from build123d import *

# Parameters (mm, degrees)
F0_R     = 9.4
F1_DEPTH = 3


with BuildPart() as f1:
    # F0 (on Front) → F1 (new body)
    with BuildSketch(Plane.XZ):
        with BuildLine():
            ThreePointArc((-5.1, -8.833459), (-3.333588, -10.15167), (-1.922689, -11.844968))
            ThreePointArc((-1.922689, -11.844968), (-0.788709, -14.298908), (-0.4, -16.974098))
            ThreePointArc((-0.4, -16.974098), (0.966541, -22.074098), (4.7, -25.807557))
            ThreePointArc((4.7, -25.807557), (8.140639, -29.248196), (9.4, -33.948196))
            ThreePointArc((9.4, -33.948196), (10.766541, -39.048196), (14.5, -42.781655))
            ThreePointArc((14.5, -42.781655), (17.940639, -46.222294), (19.2, -50.922294))
            ThreePointArc((19.2, -50.922294), (20.566541, -56.022294), (24.3, -59.755753))
            ThreePointArc((24.3, -59.755753), (27.740639, -63.196392), (29, -67.896392))
            ThreePointArc((29, -67.896392), (30.366541, -72.996392), (34.1, -76.729851))
            ThreePointArc((34.1, -76.729851), (37.540639, -80.17049), (38.8, -84.87049))
            ThreePointArc((38.8, -84.87049), (40.166541, -89.97049), (43.9, -93.703949))
            ThreePointArc((43.9, -93.703949), (47.340639, -97.144587), (48.6, -101.844587))
            ThreePointArc((48.6, -101.844587), (48.341601, -104.033451), (47.580612, -106.101974))
            ThreePointArc((47.580612, -106.101974), (51.984159, -111.72104), (58.8, -113.844587))
            Line((58.8, -113.844587), (98, -113.844587))
            ThreePointArc((98, -113.844587), (104.815841, -111.72104), (109.219388, -106.101974))
            ThreePointArc((109.219388, -106.101974), (108.458399, -104.033451), (108.2, -101.844587))
            ThreePointArc((108.2, -101.844587), (106.833459, -96.744587), (103.1, -93.011128))
            ThreePointArc((103.1, -93.011128), (99.659361, -89.57049), (98.4, -84.87049))
            ThreePointArc((98.4, -84.87049), (97.033459, -79.77049), (93.3, -76.03703))
            ThreePointArc((93.3, -76.03703), (89.859361, -72.596392), (88.6, -67.896392))
            ThreePointArc((88.6, -67.896392), (87.233459, -62.796392), (83.5, -59.062933))
            ThreePointArc((83.5, -59.062933), (80.059361, -55.622294), (78.8, -50.922294))
            ThreePointArc((78.8, -50.922294), (77.433459, -45.822294), (73.7, -42.088835))
            ThreePointArc((73.7, -42.088835), (70.259361, -38.648196), (69, -33.948196))
            ThreePointArc((69, -33.948196), (67.633459, -28.848196), (63.9, -25.114737))
            ThreePointArc((63.9, -25.114737), (60.459361, -21.674098), (59.2, -16.974098))
            ThreePointArc((59.2, -16.974098), (57.833459, -11.874098), (54.1, -8.140639))
            ThreePointArc((54.1, -8.140639), (50.659361, -4.7), (49.4, 0))
            ThreePointArc((49.4, 0), (49.658399, 2.188863), (50.419388, 4.257386))
            ThreePointArc((50.419388, 4.257386), (46.015841, 9.876453), (39.2, 12))
            Line((39.2, 12), (0, 12))
            ThreePointArc((0, 12), (-6.815841, 9.876453), (-11.219388, 4.257386))
            ThreePointArc((-11.219388, 4.257386), (-10.2, 0), (-11.219388, -4.257386))
            ThreePointArc((-11.219388, -4.257386), (-10.392305, -6), (-9.296699, -7.587582))
            ThreePointArc((-9.296699, -7.587582), (-7.12481, -7.962807), (-5.1, -8.833459))
        make_face()
        with BuildLine():
            ThreePointArc((56.877311, -89.99962), (39.988709, -82.1953), (58.4, -84.87049))
            ThreePointArc((58.4, -84.87049), (58.011291, -87.545679), (56.877311, -89.99962))
        make_face(mode=Mode.SUBTRACT)
        with Locations((39.2, -67.896392)):
            Circle(F0_R, mode=Mode.SUBTRACT)
        with Locations((58.8, -101.844587)):
            Circle(F0_R, mode=Mode.SUBTRACT)
        with Locations((78.4, -101.844587)):
            Circle(F0_R, mode=Mode.SUBTRACT)
        with BuildLine():
            ThreePointArc((78, -84.87049), (71.27519, -93.88178), (60.722689, -89.99962))
            ThreePointArc((60.722689, -89.99962), (65.92481, -75.859199), (78, -84.87049))
        make_face(mode=Mode.SUBTRACT)
        with Locations((98, -101.844587)):
            Circle(F0_R, mode=Mode.SUBTRACT)
        with Locations((88.2, -84.87049)):
            Circle(F0_R, mode=Mode.SUBTRACT)
        with Locations((58.8, -67.896392)):
            Circle(F0_R, mode=Mode.SUBTRACT)
        with Locations((78.4, -67.896392)):
            Circle(F0_R, mode=Mode.SUBTRACT)
        with Locations((29.4, -50.922294)):
            Circle(F0_R, mode=Mode.SUBTRACT)
        with Locations((49, -50.922294)):
            Circle(F0_R, mode=Mode.SUBTRACT)
        with Locations((19.6, -33.948196)):
            Circle(F0_R, mode=Mode.SUBTRACT)
        with Locations((39.2, -33.948196)):
            Circle(F0_R, mode=Mode.SUBTRACT)
        with BuildLine():
            ThreePointArc((1.922689, -11.844968), (12.47519, -7.962807), (19.2, -16.974098))
            ThreePointArc((19.2, -16.974098), (7.12481, -25.985389), (1.922689, -11.844968))
        make_face(mode=Mode.SUBTRACT)
        Circle(F0_R, mode=Mode.SUBTRACT)
        with Locations((29.4, -16.974098)):
            Circle(F0_R, mode=Mode.SUBTRACT)
        with BuildLine():
            ThreePointArc((53.7, -25.114737), (40.859361, -21.674098), (44.3, -8.833459))
            ThreePointArc((44.3, -8.833459), (57.140639, -12.274098), (53.7, -25.114737))
        make_face(mode=Mode.SUBTRACT)
        with Locations((19.6, 0)):
            Circle(F0_R, mode=Mode.SUBTRACT)
        with Locations((39.2, 0)):
            Circle(F0_R, mode=Mode.SUBTRACT)
        with Locations((68.6, -50.922294)):
            Circle(F0_R, mode=Mode.SUBTRACT)
        with Locations((58.8, -33.948196)):
            Circle(F0_R, mode=Mode.SUBTRACT)
    extrude(amount=F1_DEPTH)


solid = f1.part
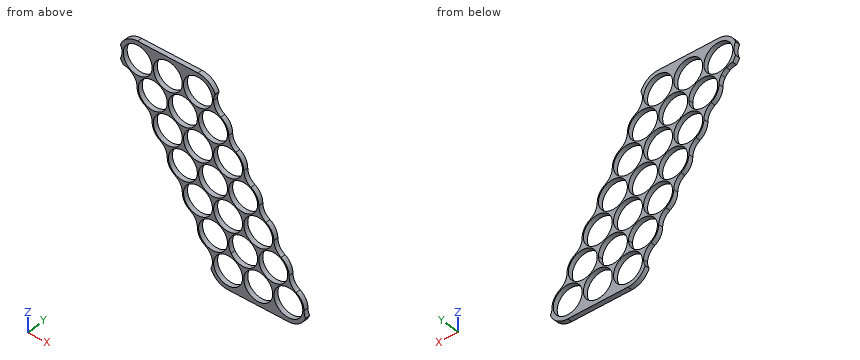
Design review of the part built by this model. Coordinates are the model's own, in mm. Coordinates: 2 decimals unless noted, no trailing zeros. Use one line per item in the form item = value.
(1) For line 1 along X through (y, z) = (-1.85, -34); line 2 along X through (y, z) = (-2.4, -12); line 3 along Z through (x, y) = (90.5, -2.2), list the stretches that pass through material, from the lowest coordinate up. Write a range as from..to.
Return value:
line_1 = 9.4..10.2, 29..29.8, 48.6..49.4, 68.2..69
line_2 = -1.82..1.82, 17.78..21.42, 37.38..41.02, 56.98..57.9
line_3 = -113.84..-107.51, -96.18..-93.98, -75.76..-73.56
(2) Consider section A-A (y = -1.25). Give the number of separate pieces and of enclosed holes in the cut face, and give its area (3 significant figures).
Return value:
separate_pieces = 1
enclosed_holes = 21
area = 1,640 mm2
(3) Clearance check with flat-ended pins moving along their axes: P1, Ø1, axis at x = 65.5, y = -1.5, coming from the +Z side; P2, Ø1, axis at y = -2, z = -80, coming from the -X side. State where each tip first meets the part, or that it passes through.
Return value:
P1 = -25.85
P2 = 37.11
